```python
from build123d import *

# Parameters (mm, degrees)
SKETCH_1_W             = 56.4
SKETCH_1_H             = 20
EXTRUDE_1_DEPTH        = 3
SKETCH_2_W             = 56.4
SKETCH_2_H             = 3
EXTRUDE_2_DEPTH        = 17
EXTRUDE_3_DEPTH        = 3
PATTERN_LINEAR_1_COUNT = 3
PATTERN_LINEAR_1_PITCH = 26.7
HOLE_WIZARD_M4_1_D     = 4.5


with BuildPart() as part:
    # 스케치1 → 보스-돌출1 (new body)
    with BuildSketch(Plane.XY):
        Rectangle(SKETCH_1_W, SKETCH_1_H)
    extrude(amount=EXTRUDE_1_DEPTH)

    # 스케치2 → 보스-돌출2 (add)
    with BuildSketch(Plane.XY.offset(3)):
        with Locations((0, 8.5)):
            Rectangle(SKETCH_2_W, SKETCH_2_H)
    extrude(amount=EXTRUDE_2_DEPTH)

    # 스케치4 → 보스-돌출3 (add)
    with BuildSketch(Plane.ZY.offset(28.2)):
        with BuildLine():
            Line((3, -10), (3, 7))
            Line((3, 7), (20, 7))
            add(Edge.make_bspline(
                [(3, -10), (5.833333333, 4.166666667), (20, 7)],
                knots=[0, 0, 0, 1, 1, 1], degree=2))
        make_face()
    extrude_3 = extrude(amount=-EXTRUDE_3_DEPTH)

    # 선형 패턴1: 보스-돌출3 ×3
    with Locations(*[(i * PATTERN_LINEAR_1_PITCH, 0, 0) for i in range(1, PATTERN_LINEAR_1_COUNT)]):
        add(extrude_3)

    # M4 여유 구멍1 (through all)
    with Locations(Plane.XY.offset(3)):
        with Locations((-13.35, 0), (13.35, 0)):
            Hole(HOLE_WIZARD_M4_1_D / 2)


solid = part.part
```
Verification items for the finished model (mm, model axes). A direction names the side the tool comes from. Coordinates: 2 decimals unless noted, no trailing zeros. Write each loop counter-clockwise with the first axis right and the second up, starting at its lowest first coordinate (ties: lowest second). Pieces come first, ordered by that corner, then holes. Notation, with made-up numbers: M -25,36.5 L 16,36.5 A19 ccw 16,45.5 Z; hole C 82.25,40 d2. An arc over 180 degrees is marked long. Answer as a JSON object with one key per item and string values. Group by question number.
(1) Cross-section at C-C, the plane y = 1.25. State how many separate pieces and enclosed holes the cut face has, and give its area (3 significant figures).
(2) Material ranges on line 1 (X direction, y = 6.25, z = 8.75); line 2 (Y direction, x = -13.35, z = 0.75); line 3 (Z direction, x = 16.5, y = -3), recorded low to high.
(3) Cross-section at A-A, the plane x = -13.35. Record the cut outline in (y, z).
(4) Tool access check on faces 4 (the face through (-15.496, 0.676, 1.479)), 5 (the face through (-14, 7, 11)). Record the directions out of +Z, -Z, +X, -X, +Y, -Y that give a thin tool (end or side, any length) a straight path to the whole face; none if there is none.
(5) Release check for a two-part mould opening along X. For faces 1 (the face through (15.598, 0.099, 1.479)), 2 (the face through (28.2, 5, 8)), 3 (the face through (-28.2, 5, 8)) record: +X half, -X half, draft (parallel to the pull), parting line (faces both ways), or undercut.
(6) Cross-section at B-B, the plane x = 3. Record the cut outline in (y, z), and give its area (3 significant figures).
(7) Gauge pin test, flat ends, axial feed: pin 1 (1.5 mm diameter, centred on x = -20.5, z = 14.5, fed in from -Y); pin 2 (8 mm diameter, centred on x = 19.5, y = 0, fed in from +Z). Record the tip position at first contact, or that the pin passes through.
Reply:
{
 "1": {"separate pieces": "3", "enclosed holes": "0", "area": "197 mm²"},
 "2": {"line 1": "-28.2 to -25.2, -1.5 to 1.5, 25.2 to 28.2", "line 2": "-10 to -2.25, 2.25 to 10", "line 3": "0 to 3"},
 "3": {"outline": "M -10,0 L -2.25,0 L -2.25,3 L -10,3 Z; M 2.25,0 L 10,0 L 10,20 L 7,20 L 7,3 L 2.25,3 Z"},
 "4": {"face 4": "+Z, -Z", "face 5": "+Z, -Y"},
 "5": {"face 1": "undercut", "face 2": "+X half", "face 3": "-X half"},
 "6": {"outline": "M -10,0 L 10,0 L 10,20 L 7,20 L 7,3 L -10,3 Z", "area": "111 mm²"},
 "7": {"pin 1": "y = 7", "pin 2": "z = 3"}
}
